Check sheet for the modelled part. Datum: model origin and axes. Units: mm. Face numbers are marked on the shaded views. Coordinates: 2 decimals unless noted, no trailing zeros. Order: outer loops, then holes, each group sorted by start corner. A loop starts at its lowest first (then second) coordinate and runs counter-clockwise, first axis right, second up. Notation, with made-up numbers: (19, -20) -> (78, -20) arc R18 cw to (78, 15) -> close; hole circle Ø8 at (31, -20.75). An arc over 180 degrees is marked (long way). Put each result on its own line as item: value. Start each with the question number.
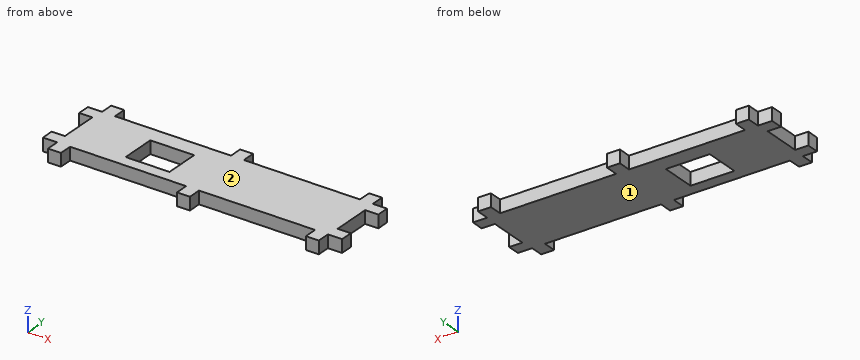
```python
from build123d import *

# Parameters (mm, degrees)
SKETCH1_W           = 116
SKETCH1_H           = 12.3
BOSS_EXTRUDE1_DEPTH = 5
SKETCH2_W           = 5
SKETCH2_H           = 5
BOSS_EXTRUDE2_DEPTH = 5
SKETCH3_W           = 17
SKETCH3_H           = 13.5
CUT_EXTRUDE1_DEPTH  = 6
SKETCH4_W           = 5
SKETCH4_H           = 15.1
CUT_EXTRUDE2_DEPTH  = 5.1


with BuildPart() as part:
    # Sketch1 → Boss-Extrude1 (new body)
    with BuildSketch(Plane.XY):
        Rectangle(SKETCH1_W, SKETCH1_H)
    extrude(amount=BOSS_EXTRUDE1_DEPTH)

    # Sketch2 → Boss-Extrude2 (add)
    with BuildSketch(Plane.XZ.offset(6.15)):
        with Locations((-50, 2.5)):
            Rectangle(SKETCH2_W, SKETCH2_H)
        with Locations((0, 2.5)):
            Rectangle(SKETCH2_W, SKETCH2_H)
        with Locations((50, 2.5)):
            Rectangle(SKETCH2_W, SKETCH2_H)
    extrude(amount=BOSS_EXTRUDE2_DEPTH)

    # Mirror1: part across plane


with BuildPart() as part_1:
    add(part.part)
    add(part.part.mirror(Plane(origin=(-58, 6.15, 5), x_dir=(0, 0, 1), z_dir=(0, -1, 0))))

    # Sketch3 → Cut-Extrude1 (cut, through all)
    with BuildSketch(Plane.XY.offset(5)):
        with Locations((-20.7, 5.2)):
            Rectangle(SKETCH3_W, SKETCH3_H)
    extrude(amount=-CUT_EXTRUDE1_DEPTH, mode=Mode.SUBTRACT)

    # Sketch4 → Cut-Extrude2 (cut)
    with BuildSketch(Plane.ZY.offset(58)):
        with Locations((2.5, 6.15)):
            Rectangle(SKETCH4_W, SKETCH4_H)
    cut_extrude2 = extrude(amount=-CUT_EXTRUDE2_DEPTH, mode=Mode.SUBTRACT)

    # Mirror2: Cut-Extrude2 across plane
    add(cut_extrude2.mirror(Plane(origin=(0, 0, 0), x_dir=(0, 0, 1), z_dir=(1, 0, 0))), mode=Mode.SUBTRACT)


solid = part_1.part
```
1) Sectioned sample at A-A (y = 7). Record the boundary of the cut face in (x, z).
2) Mould release check, pull along Z, two halves, no side actions. Record for the marked faces 1 and 2: +Z half, -Z half, draft (parallel to the pull), parting line (faces both ways), or undercut.
3) Sectioned sample at B-B (y = 21). Record the boundary of the cut face in (x, z).
4) Scan lines: line 1 along X through (y, z) = (0, 0.6); line 2 along X through (y, z) = (20.5, 4.25); line 3 along Y through (x, z) = (-53, 4.65). Record each from-to range of solid material in increasing order. Write a range as [from, to].
5) Gauge pin test, flat ends, axial feed: pin 1 (1 mm diameter, centred on x = 29, z = 4, fed in from -Y); pin 2 (2.5 mm diameter, centred on x = -22, z = 1.5, fed in from +Y); pin 3 (2.5 mm diameter, centred on y = 22, z = 3, fed in from -X). Record the tip position at first contact, or that the pin passes through.
6) Sectioned sample at C-C (x = 38). Record the boundary of the cut face in (y, z).
Entries:
1. outline: (-52.9, 0) -> (-29.2, 0) -> (-29.2, 5) -> (-52.9, 5) -> close; (-12.2, 0) -> (52.9, 0) -> (52.9, 5) -> (-12.2, 5) -> close
2. face 1: -Z half
2. face 2: +Z half
3. outline: (-52.5, 0) -> (-47.5, 0) -> (-47.5, 5) -> (-52.5, 5) -> close; (-2.5, 0) -> (2.5, 0) -> (2.5, 5) -> (-2.5, 5) -> close; (47.5, 0) -> (52.5, 0) -> (52.5, 5) -> (47.5, 5) -> close
4. line 1: x = [-52.9, -29.2], [-12.2, 52.9]
4. line 2: x = [-52.5, -47.5], [-2.5, 2.5], [47.5, 52.5]
4. line 3: y = [-6.15, -1.4], [13.7, 18.45]
5. pin 1: stops at y = -6.15
5. pin 2: stops at y = 18.45
5. pin 3: stops at x = -52.5
6. outline: (-6.15, 0) -> (18.45, 0) -> (18.45, 5) -> (-6.15, 5) -> close
